```python
from build123d import *

# Parameters (mm, degrees)
F1_DEPTH = 50.8
F3_D     = 2.2606
F4_R     = 2.54
F5_R     = 2.54


with BuildPart() as f1:
    # F0 (on Right) → F1 (new body)
    with BuildSketch(Plane.YZ):
        Polygon((-2.3067509514, -0.331221791), (-2.3067509514, 7.168778209), (-6.3067509514, 7.168778209), (-6.3067509514, -11.055721791), (0.9745705689, -11.055721791), (0.9431016669, -0.3002708691), align=None)
    extrude(amount=F1_DEPTH)

    # F3 (through all)
    with Locations(Plane.XZ.offset(6.3067509514)):
        with Locations((12.7, -5.721721791), (38.1, -5.721721791)):
            Hole(F3_D / 2)

    # F4
    f4_edges = [f1.edges().sort_by_distance(p)[0] for p in [
        (50.8, -4.306751, 7.168778),
    ]]
    fillet(f4_edges, radius=F4_R)

    # F5
    f5_edges = [f1.edges().sort_by_distance(p)[0] for p in [
        (0, -4.306751, 7.168778),
    ]]
    fillet(f5_edges, radius=F5_R)


solid = f1.part
```
The listing builds one solid part. Answer for the finished solid, in the listing's coordinates (mm). Coordinates: 2 decimals unless noted, no trailing zeros. Loops run counter-clockwise (first coordinate to the right, second up) from the corner with the lowest first, then second, coordinate; pieces in that order, holes last. Notation, with made-up numbers: M -27,-12 L 2,-12 A17 cw 2,5 Z; hole C 38,71.25 d2. An arc over 180 degrees is marked long. Answer as CSV lines item,"result". Start each with the question number.
(1) The part is cut by section B-B (y = -0.5). Give the vertices of the cut face in (x, z), and give its area (3 significant figures).
(2) The part is cut by section C-C (x = 7.5). Give the vertices of the cut face in (y, z), and give its area (3 significant figures).
(3) The part is cut by section A-A (x = 12.7). Give the vertices of the cut face in (y, z).
(4) The part is cut by section D-D (z = 6.25). Give the vertices of the cut face in (x, y), and give its area (3 significant figures).
(5) Given pin 1 (6 mm diameter, centred on x = 43.5, z = -4, fed in from +Y); pin 2 (8.5 mm diameter, centred on x = 19, z = 4.5, fed in from +Y); pin 3 (2 mm diameter, centred on x = 38.1, z = -5.72, fed in from +Y), each flat-ended and moving along its own axis, determine where each tip first touches the part or whether it passes through.
(6) Find the intervals of material crossed by L1, parallel to Z at x = 12.7, y = -0.25; L2, parallel to Z at x = 12.7, y = -3.5; L3, parallel to X at y = -0.75, z = -6.75, in increasing order. Write a range as [from, to].
Determined:
1,outline,"M 0,-11.06 L 50.8,-11.06 L 50.8,-0.31 L 0,-0.31 Z; hole C 12.7,-5.72 d2.26; hole C 38.1,-5.72 d2.26"
1,area,"538 mm2"
2,outline,"M -6.31,-11.06 L 0.97,-11.06 L 0.94,-0.3 L -2.31,-0.33 L -2.31,7.17 L -6.31,7.17 Z"
2,area,"108 mm2"
3,outline,"M -6.31,-11.06 L 0.97,-11.06 L 0.96,-6.85 L -6.31,-6.85 Z; M -6.31,-4.59 L 0.96,-4.59 L 0.94,-0.3 L -2.31,-0.33 L -2.31,7.17 L -6.31,7.17 Z"
4,outline,"M 0.58,-6.31 L 50.22,-6.31 L 50.22,-2.31 L 0.58,-2.31 Z"
4,area,"199 mm2"
5,pin 1,"y = 0.96"
5,pin 2,"y = -2.31"
5,pin 3,"through"
6,L1,"[-11.06, -6.85], [-4.59, -0.31]"
6,L2,"[-11.06, -6.85], [-4.59, 7.17]"
6,L3,"[0, 12.23], [13.17, 37.63], [38.57, 50.8]"
